from build123d import *

# Parameters (mm, degrees)
F0_W     = 50
F0_H     = 20
F1_DEPTH = 2
F2_W     = 1.5
F2_H     = 20
F3_DEPTH = 10
F4_W     = 20
F4_H     = 20
F5_DEPTH = 2
F6_SIZE  = 1


with BuildPart() as f1:
    # F0 (on Top) → F1 (new body)
    with BuildSketch(Plane.XY):
        Rectangle(F0_W, F0_H)
    extrude(amount=F1_DEPTH)

    # F2 (on face) → F3 (join)
    with BuildSketch(Plane.XY.offset(2)):
        with Locations((-24.25, 0)):
            Rectangle(F2_W, F2_H)
        with Locations((24.25, 0)):
            Rectangle(F2_W, F2_H)
    extrude(amount=F3_DEPTH)

    # F4 (on face) → F5 (join)
    with BuildSketch(Plane.XY.offset(12)):
        with Locations((-33.5, 0)):
            Rectangle(F4_W, F4_H)
        with Locations((33.5, 0)):
            Rectangle(F4_W, F4_H)
    extrude(amount=F5_DEPTH)

    # F6
    f6_edges = [f1.edges().sort_by_distance(p)[0] for p in [
        (-25, 0, 0),
        (25, 0, 0),
        (-43.5, 0, 12),
        (43.5, 0, 12),
        (34.25, -10, 12),
        (34.25, 10, 12),
        (-34.25, 10, 12),
    ]]
    chamfer(f6_edges, length=F6_SIZE)


solid = f1.part
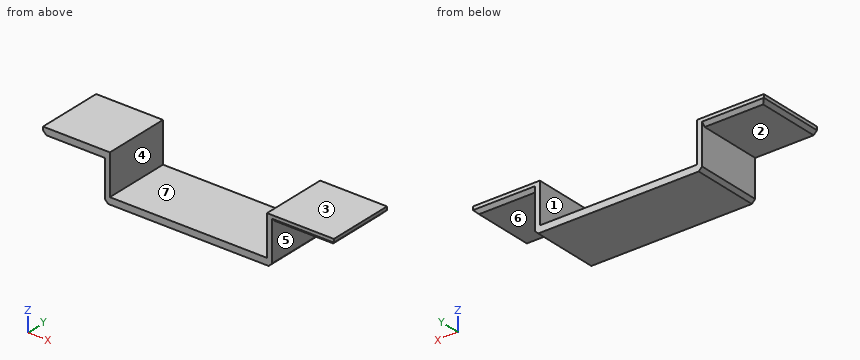
Build history of the part. All positions in model axes, mm. Face numbers are marked on the shaded views. A direction names the side the tool comes from. Coordinates: 2 decimals unless noted, no trailing zeros. Order: outer loops, then holes, each group sorted by start corner. A loop starts at its lowest first (then second) coordinate and runs counter-clockwise, first axis right, second up. Notation, with made-up numbers: (-10.5, 80) - (0.5, 80) arc R19 ccw to (0.5, 110) - close; hole circle Ø6 at (81, 50.5). An arc over 180 degrees is marked (long way). Write each question's results on one line, items separated by ' | '. Start each with the question number.
Item 1: Tool access for the marked faces 1, 2 and 3: list every direction of +Z, -Z, +X, -X, +Y, -Y with a clear straight run to the whole face (end or side of a thin tool).
Item 2: Wall check: probe 1 along X at (y, z) = (-3, 2.5); probe 2 along Z at (x, y) = (17.5, -5.75); probe 3 along Z at (x, y) = (40.5, -8.5). Give the ranges that are in metal, low to high. Write a range as [from, to].
Item 3: Band-saw the part on B-B on x = 27.5. Write the cut outline in (y, z), and give its area (3 significant figures).
Item 4: Band-saw the part on C-C on y = -4.5. Write the cut outline in (x, z), and give its area (3 significant figures).
Item 5: Flat gauge pins, fed straight in: pin 1 (3 mm diameter, centred on y = -5.5, z = 3, fed in from -X); pin 2 (6 mm diameter, centred on y = -3.5, z = 7, fed in from +X); pin 3 (5 mm diameter, centred on x = -35, y = -3, fed in from -Z); pin 4 (8 mm diameter, centred on x = 13, z = 8.5, fed in from -Y). Where does each tip first touch, or does it go through?
Item 6: Mould opens along X. For the marked faces 4, 5, 6 and 7 say: released by +X, released by -X, zero draft, split by the parting line, or undercut.
Item 7: Band-saw the part on A-A on z = 11. Write the cut outline in (x, y).
Numbers:
1) face 1: +Z, +Y, -Y | face 2: -Z, -X, +Y, -Y | face 3: +Z, +X, -X, +Y, -Y
2) probe 1: [-25, -23.5], [23.5, 25] | probe 2: [0, 2] | probe 3: [12, 14]
3) outline: (-10, 13) - (-9, 12) - (9, 12) - (10, 13) - (10, 14) - (-10, 14) - close | area: 39.0 mm^2
4) outline: (-43.5, 13) - (-42.5, 12) - (-25, 12) - (-25, 1) - (-24, 0) - (24, 0) - (25, 1) - (25, 12) - (42.5, 12) - (43.5, 13) - (43.5, 14) - (23.5, 14) - (23.5, 2) - (-23.5, 2) - (-23.5, 14) - (-43.5, 14) - close | area: 208 mm^2
5) pin 1: x = -25 | pin 2: x = 25 | pin 3: z = 12 | pin 4: through
6) face 4: undercut | face 5: released by +X | face 6: zero draft | face 7: undercut
7) outline: (-25, -10) - (-23.5, -10) - (-23.5, 10) - (-25, 10) - close; (23.5, -10) - (25, -10) - (25, 10) - (23.5, 10) - close
